The model under review builds one solid part; all positions refer to its coordinate system, in mm. Round coordinates to 2 decimals unless told otherwise and drop trailing zeros. Write each loop counter-clockwise with the first axis right and the second up, starting at its lowest first coordinate (ties: lowest second). Pieces come first, ordered by that corner, then holes. Notation, with made-up numbers: (-33.75, 57.5) - (15.25, 57.5) arc R14 cw to (15.25, 74.5) - close; hole circle Ø2 at (14.25, 75.5). An arc over 180 degrees is marked (long way). Return JSON: item names as keys, results as strings.
from build123d import *

# Parameters (mm, degrees)
SKETCH1_R           = 4.318
BOSS_EXTRUDE1_DEPTH = 1.191006


with BuildPart() as part:
    # Sketch1 → Boss-Extrude1 (new body)
    with BuildSketch(Plane(origin=(0, 0, 0), x_dir=(1, 0, 0), z_dir=(0, 1, 0))):
        Polygon((7.332348419, 0), (3.666174209, 6.35), (-3.666174209, 6.35), (-7.332348419, 0), (-3.666174209, -6.35), (3.666174209, -6.35), align=None)
        with Locations(Location((0, 0, 0), (0, 0, 270))):
            Circle(SKETCH1_R, mode=Mode.SUBTRACT)
    extrude(amount=BOSS_EXTRUDE1_DEPTH)

    # Sketch2 → Cut-Revolve1 (revolve, cut)
    with BuildSketch(Plane.XY, mode=Mode.PRIVATE) as cut_revolve1_sk:
        Polygon((4.7625, 1.191006), (4.318, 0.794004), (4.7625, 0.397002), (4.318, 0), (0, 0), (0, 1.191006), align=None)
    revolve(cut_revolve1_sk.sketch.rotate(Axis((0, 1.191006, 0), (0, -1, 0)), 180), axis=Axis((0, 1.191006, 0), (0, -1, 0)), mode=Mode.SUBTRACT)


solid = part.part
(1) Wall thickness on line 1 (Z direction, x = -3.25, y = 1.1); line 2 (X direction, y = 1.05, z = 2.25); line 3 (X direction, y = 0.95, z = 3): over which ranges is each line inside the solid? List them lowest first.
Filled in:
{"line 1": "z = -6.35 to -3.34, 3.34 to 6.35", "line 2": "x = -6.03 to -4.02, 4.02 to 6.03", "line 3": "x = -5.6 to -3.34, 3.34 to 5.6"}
(2) Add section B-B (x = 0). Write out the cut boundary in (y, z), plus the area to 3 significant figures.
Filled in:
{"outline": "(0, -6.35) - (1.19, -6.35) - (1.19, -4.76) - (0.79, -4.32) - (0.4, -4.76) - (0, -4.32) - close; (0, 4.32) - (0.4, 4.76) - (0.79, 4.32) - (1.19, 4.76) - (1.19, 6.35) - (0, 6.35) - close", "area": "4.31 mm2"}
(3) Add section C-C (z = 5.25). Write out the cut boundary in (x, y), plus the area to 3 significant figures.
Filled in:
{"outline": "(-4.3, 0) - (4.3, 0) - (4.3, 1.19) - (-4.3, 1.19) - close", "area": "10.2 mm2"}
(4) Add section A-A (y = 0.95). Write out the cut boundary in (x, z).
Filled in:
{"outline": "(-7.33, 0) - (-3.67, -6.35) - (3.67, -6.35) - (7.33, 0) - (3.67, 6.35) - (-3.67, 6.35) - close; hole circle Ø8.99 at (0, 0)"}
(5) Add section D-D (x = -6.5). Write out the cut boundary in (y, z).
Filled in:
{"outline": "(0, -1.44) - (1.19, -1.44) - (1.19, 1.44) - (0, 1.44) - close"}
